Check sheet for the modelled part. Datum: model origin and axes. Units: mm. Face numbers are marked on the shaded views. Coordinates: 2 decimals unless noted, no trailing zeros. Loops run counter-clockwise (first coordinate to the right, second up) from the corner with the lowest first, then second, coordinate; pieces in that order, holes last. Notation, with made-up numbers: (1, -29) - (44, -29) arc R32 ccw to (44, 8) - close; hole circle Ø5 at (68, -31.75). An arc over 180 degrees is marked (long way). Write each question's results on one line, items separated by ' | '. Start each with the question number.
1. Cross-section at A-A (z = 7.5). Record the cut outline in (x, y).
2. Thickness scan on line 1 (Y direction, x = -18, z = 17.5); line 2 (X direction, y = 0, z = -17); line 3 (Y direction, x = 0, z = -17.5). Record the ranges inside material, lowest first. Write a range as [from, to].
3. Gauge pin test, flat ends, axial feed: P1, Ø3, axis at x = -26.5, y = -2.5, coming from the +Z side; P2, Ø4, axis at y = -2, z = -1, coming from the +X side. Record the tip position at first contact, or that the pin passes through.
4. Draft check along Y on the marked faces 1, 2, 3 and 4. Enter one of: released by +Y, released by -Y, zero draft, split by the parting line, or undercut.
5. Cross-section at C-C (z = -13). Record the cut outline in (x, y).
6. Cross-section at B-B (x = 14). Give the number of separate pieces and of enclosed holes in the cut face, and give its area (3 significant figures).
```python
from build123d import *

# Parameters (mm, degrees)
BOSS_EXTRUDE1_DEPTH     = 31
SKETCH2_R               = 18
BOSS_EXTRUDE2_DEPTH     = 1
SKETCH3_R               = 16
CUT_EXTRUDE1_DEPTH      = 73.520686704
CUT_EXTRUDE2_DEPTH      = 2
SKETCH5_R               = 3.5
CUT_EXTRUDE3_DEPTH      = 73.520686704
SKETCH6_W               = 3
SKETCH6_H               = 48
LPATTERN2_COUNT         = 9
LPATTERN2_PITCH         = 6
MIRROR1_COPY_1_SKETCH_W = 3
MIRROR1_COPY_1_SKETCH_H = 48
MIRROR1_COPY_2_SKETCH_W = 3
MIRROR1_COPY_2_SKETCH_H = 48
MIRROR1_COPY_3_SKETCH_W = 3
MIRROR1_COPY_3_SKETCH_H = 48
MIRROR1_COPY_4_SKETCH_W = 3
MIRROR1_COPY_4_SKETCH_H = 48
MIRROR1_COPY_5_SKETCH_W = 3
MIRROR1_COPY_5_SKETCH_H = 48
MIRROR1_COPY_6_SKETCH_W = 3
MIRROR1_COPY_6_SKETCH_H = 48
MIRROR1_COPY_7_SKETCH_W = 3
MIRROR1_COPY_7_SKETCH_H = 48
MIRROR1_COPY_8_SKETCH_W = 3
MIRROR1_COPY_8_SKETCH_H = 48
SKETCH8_W               = 48
SKETCH8_H               = 3
LPATTERN3_COUNT         = 9
LPATTERN3_PITCH         = 6
MIRROR2_COPY_1_SKETCH_W = 48
MIRROR2_COPY_1_SKETCH_H = 3
MIRROR2_COPY_2_SKETCH_W = 48
MIRROR2_COPY_2_SKETCH_H = 3
MIRROR2_COPY_3_SKETCH_W = 48
MIRROR2_COPY_3_SKETCH_H = 3
MIRROR2_COPY_4_SKETCH_W = 48
MIRROR2_COPY_4_SKETCH_H = 3
MIRROR2_COPY_5_SKETCH_W = 48
MIRROR2_COPY_5_SKETCH_H = 3
MIRROR2_COPY_6_SKETCH_W = 48
MIRROR2_COPY_6_SKETCH_H = 3
MIRROR2_COPY_7_SKETCH_W = 48
MIRROR2_COPY_7_SKETCH_H = 3
MIRROR2_COPY_8_SKETCH_W = 48
MIRROR2_COPY_8_SKETCH_H = 3


with BuildPart() as part:
    # Sketch1 → Boss-Extrude1 (new, symmetric)
    with BuildSketch(Plane.XY):
        with BuildLine():
            Line((18, 22.5), (-24, 22.5))
            ThreePointArc((-24, 22.5), (-26.828427125, 21.328427125), (-28, 18.5))
            Line((-28, 18.5), (-28, -18.5))
            ThreePointArc((-28, -18.5), (-26.828427125, -21.328427125), (-24, -22.5))
            Line((-24, -22.5), (18, -22.5))
            ThreePointArc((18, -22.5), (20.828427125, -21.328427125), (22, -18.5))
            Line((22, -18.5), (22, 18.5))
            ThreePointArc((22, 18.5), (20.828427125, 21.328427125), (18, 22.5))
        make_face()
    extrude(amount=BOSS_EXTRUDE1_DEPTH, both=True)

    # Sketch2 → Boss-Extrude2 (add, symmetric)
    with BuildSketch(Plane.XY.offset(31)):
        with Locations(Location((0, 0, 0), (0, 0, 180))):
            Circle(SKETCH2_R)
    extrude(amount=BOSS_EXTRUDE2_DEPTH, both=True)

    # Sketch3 → Cut-Extrude1 (cut, through all)
    with BuildSketch(Plane.XY.offset(32)):
        Circle(SKETCH3_R)
    extrude(amount=-CUT_EXTRUDE1_DEPTH, mode=Mode.SUBTRACT)

    # Sketch4 → Cut-Extrude2 (cut)
    with BuildSketch(Plane(origin=(0, 0, -31), x_dir=(-1, 0, 0), z_dir=(0, 0, -1))):
        with BuildLine():
            Line((12.872380115, 2), (12.872380115, -2))
            Line((12.872380115, -2), (22.61, -2))
            ThreePointArc((22.61, -2), (24.657927917, -0.354015138), (23.490928495, 2))
            Line((23.490928495, 2), (12.872380115, 2))
        make_face()
    extrude(amount=-CUT_EXTRUDE2_DEPTH, mode=Mode.SUBTRACT)

    # Sketch5 → Cut-Extrude3 (cut, through all)
    with BuildSketch(Plane(origin=(0, 0, -31), x_dir=(-1, 0, 0), z_dir=(0, 0, -1))):
        with Locations((-16.263455967, 16.263455967)):
            Circle(SKETCH5_R)
        with Locations((16.263455967, 16.263455967)):
            Circle(SKETCH5_R)
        with Locations((16.263455967, -16.263455967)):
            Circle(SKETCH5_R)
        with Locations((-16.263455967, -16.263455967)):
            Circle(SKETCH5_R)
    extrude(amount=-CUT_EXTRUDE3_DEPTH, mode=Mode.SUBTRACT)

    # Sketch6 → Cut-Revolve1 (revolve, cut)
    with BuildSketch(Plane(origin=(-3, 0, 0), x_dir=(0, 0, -1), z_dir=(1, 0, 0))):
        with Locations((25.5, 42.5)):
            Rectangle(SKETCH6_W, SKETCH6_H)
    cut_revolve1 = revolve(axis=Axis((-3, 66.5, -24), (0, 0, -1)), mode=Mode.SUBTRACT)

    # LPattern2: Cut-Revolve1 ×9
    with Locations(*[(0, 0, i * LPATTERN2_PITCH) for i in range(1, LPATTERN2_COUNT)]):
        add(cut_revolve1, mode=Mode.SUBTRACT)

    # Mirror1: Cut-Revolve1 across plane
    add(cut_revolve1.mirror(Plane.ZX), mode=Mode.SUBTRACT)

    # Mirror1 copy 1 sketch → Mirror1 copy 1 (revolve, cut)
    with BuildSketch(Plane(origin=(-3, 0, 6), x_dir=(0, 0, -1), z_dir=(1, 0, 0))):
        with Locations((25.5, -42.5)):
            Rectangle(MIRROR1_COPY_1_SKETCH_W, MIRROR1_COPY_1_SKETCH_H)
    revolve(axis=Axis((-3, -66.5, -18), (0, 0, 1)), mode=Mode.SUBTRACT)

    # Mirror1 copy 2 sketch → Mirror1 copy 2 (revolve, cut)
    with BuildSketch(Plane(origin=(-3, 0, 12), x_dir=(0, 0, -1), z_dir=(1, 0, 0))):
        with Locations((25.5, -42.5)):
            Rectangle(MIRROR1_COPY_2_SKETCH_W, MIRROR1_COPY_2_SKETCH_H)
    revolve(axis=Axis((-3, -66.5, -12), (0, 0, 1)), mode=Mode.SUBTRACT)

    # Mirror1 copy 3 sketch → Mirror1 copy 3 (revolve, cut)
    with BuildSketch(Plane(origin=(-3, 0, 18), x_dir=(0, 0, -1), z_dir=(1, 0, 0))):
        with Locations((25.5, -42.5)):
            Rectangle(MIRROR1_COPY_3_SKETCH_W, MIRROR1_COPY_3_SKETCH_H)
    revolve(axis=Axis((-3, -66.5, -6), (0, 0, 1)), mode=Mode.SUBTRACT)

    # Mirror1 copy 4 sketch → Mirror1 copy 4 (revolve, cut)
    with BuildSketch(Plane(origin=(-3, 0, 24), x_dir=(0, 0, -1), z_dir=(1, 0, 0))):
        with Locations((25.5, -42.5)):
            Rectangle(MIRROR1_COPY_4_SKETCH_W, MIRROR1_COPY_4_SKETCH_H)
    revolve(axis=Axis((-3, -66.5, 0), (0, 0, 1)), mode=Mode.SUBTRACT)

    # Mirror1 copy 5 sketch → Mirror1 copy 5 (revolve, cut)
    with BuildSketch(Plane(origin=(-3, 0, 30), x_dir=(0, 0, -1), z_dir=(1, 0, 0))):
        with Locations((25.5, -42.5)):
            Rectangle(MIRROR1_COPY_5_SKETCH_W, MIRROR1_COPY_5_SKETCH_H)
    revolve(axis=Axis((-3, -66.5, 6), (0, 0, 1)), mode=Mode.SUBTRACT)

    # Mirror1 copy 6 sketch → Mirror1 copy 6 (revolve, cut)
    with BuildSketch(Plane(origin=(-3, 0, 36), x_dir=(0, 0, -1), z_dir=(1, 0, 0))):
        with Locations((25.5, -42.5)):
            Rectangle(MIRROR1_COPY_6_SKETCH_W, MIRROR1_COPY_6_SKETCH_H)
    revolve(axis=Axis((-3, -66.5, 12), (0, 0, 1)), mode=Mode.SUBTRACT)

    # Mirror1 copy 7 sketch → Mirror1 copy 7 (revolve, cut)
    with BuildSketch(Plane(origin=(-3, 0, 42), x_dir=(0, 0, -1), z_dir=(1, 0, 0))):
        with Locations((25.5, -42.5)):
            Rectangle(MIRROR1_COPY_7_SKETCH_W, MIRROR1_COPY_7_SKETCH_H)
    revolve(axis=Axis((-3, -66.5, 18), (0, 0, 1)), mode=Mode.SUBTRACT)

    # Mirror1 copy 8 sketch → Mirror1 copy 8 (revolve, cut)
    with BuildSketch(Plane(origin=(-3, 0, 48), x_dir=(0, 0, -1), z_dir=(1, 0, 0))):
        with Locations((25.5, -42.5)):
            Rectangle(MIRROR1_COPY_8_SKETCH_W, MIRROR1_COPY_8_SKETCH_H)
    revolve(axis=Axis((-3, -66.5, 24), (0, 0, 1)), mode=Mode.SUBTRACT)

    # Sketch8 → Cut-Revolve2 (revolve, cut)
    with BuildSketch(Plane(origin=(0, 0, 0), x_dir=(1, 0, 0), z_dir=(0, 1, 0))):
        with Locations((-48, 25.5)):
            Rectangle(SKETCH8_W, SKETCH8_H)
    cut_revolve2 = revolve(axis=Axis((-72, 0, -27), (0, 0, 1)), mode=Mode.SUBTRACT)

    # LPattern3: Cut-Revolve2 ×9
    with Locations(*[(0, 0, i * LPATTERN3_PITCH) for i in range(1, LPATTERN3_COUNT)]):
        add(cut_revolve2, mode=Mode.SUBTRACT)

    # Mirror2: Cut-Revolve2 across plane
    add(cut_revolve2.mirror(Plane(origin=(-3, 0, 0), x_dir=(0, 0, 1), z_dir=(1, 0, 0))), mode=Mode.SUBTRACT)

    # Mirror2 copy 1 sketch → Mirror2 copy 1 (revolve, cut)
    with BuildSketch(Plane(origin=(-6, 0, 6), x_dir=(-1, 0, 0), z_dir=(0, 1, 0))):
        with Locations((-48, -25.5)):
            Rectangle(MIRROR2_COPY_1_SKETCH_W, MIRROR2_COPY_1_SKETCH_H)
    revolve(axis=Axis((66, 0, -21), (0, 0, -1)), mode=Mode.SUBTRACT)

    # Mirror2 copy 2 sketch → Mirror2 copy 2 (revolve, cut)
    with BuildSketch(Plane(origin=(-6, 0, 12), x_dir=(-1, 0, 0), z_dir=(0, 1, 0))):
        with Locations((-48, -25.5)):
            Rectangle(MIRROR2_COPY_2_SKETCH_W, MIRROR2_COPY_2_SKETCH_H)
    revolve(axis=Axis((66, 0, -15), (0, 0, -1)), mode=Mode.SUBTRACT)

    # Mirror2 copy 3 sketch → Mirror2 copy 3 (revolve, cut)
    with BuildSketch(Plane(origin=(-6, 0, 18), x_dir=(-1, 0, 0), z_dir=(0, 1, 0))):
        with Locations((-48, -25.5)):
            Rectangle(MIRROR2_COPY_3_SKETCH_W, MIRROR2_COPY_3_SKETCH_H)
    revolve(axis=Axis((66, 0, -9), (0, 0, -1)), mode=Mode.SUBTRACT)

    # Mirror2 copy 4 sketch → Mirror2 copy 4 (revolve, cut)
    with BuildSketch(Plane(origin=(-6, 0, 24), x_dir=(-1, 0, 0), z_dir=(0, 1, 0))):
        with Locations((-48, -25.5)):
            Rectangle(MIRROR2_COPY_4_SKETCH_W, MIRROR2_COPY_4_SKETCH_H)
    revolve(axis=Axis((66, 0, -3), (0, 0, -1)), mode=Mode.SUBTRACT)

    # Mirror2 copy 5 sketch → Mirror2 copy 5 (revolve, cut)
    with BuildSketch(Plane(origin=(-6, 0, 30), x_dir=(-1, 0, 0), z_dir=(0, 1, 0))):
        with Locations((-48, -25.5)):
            Rectangle(MIRROR2_COPY_5_SKETCH_W, MIRROR2_COPY_5_SKETCH_H)
    revolve(axis=Axis((66, 0, 3), (0, 0, -1)), mode=Mode.SUBTRACT)

    # Mirror2 copy 6 sketch → Mirror2 copy 6 (revolve, cut)
    with BuildSketch(Plane(origin=(-6, 0, 36), x_dir=(-1, 0, 0), z_dir=(0, 1, 0))):
        with Locations((-48, -25.5)):
            Rectangle(MIRROR2_COPY_6_SKETCH_W, MIRROR2_COPY_6_SKETCH_H)
    revolve(axis=Axis((66, 0, 9), (0, 0, -1)), mode=Mode.SUBTRACT)

    # Mirror2 copy 7 sketch → Mirror2 copy 7 (revolve, cut)
    with BuildSketch(Plane(origin=(-6, 0, 42), x_dir=(-1, 0, 0), z_dir=(0, 1, 0))):
        with Locations((-48, -25.5)):
            Rectangle(MIRROR2_COPY_7_SKETCH_W, MIRROR2_COPY_7_SKETCH_H)
    revolve(axis=Axis((66, 0, 15), (0, 0, -1)), mode=Mode.SUBTRACT)

    # Mirror2 copy 8 sketch → Mirror2 copy 8 (revolve, cut)
    with BuildSketch(Plane(origin=(-6, 0, 48), x_dir=(-1, 0, 0), z_dir=(0, 1, 0))):
        with Locations((-48, -25.5)):
            Rectangle(MIRROR2_COPY_8_SKETCH_W, MIRROR2_COPY_8_SKETCH_H)
    revolve(axis=Axis((66, 0, 21), (0, 0, -1)), mode=Mode.SUBTRACT)


solid = part.part
```
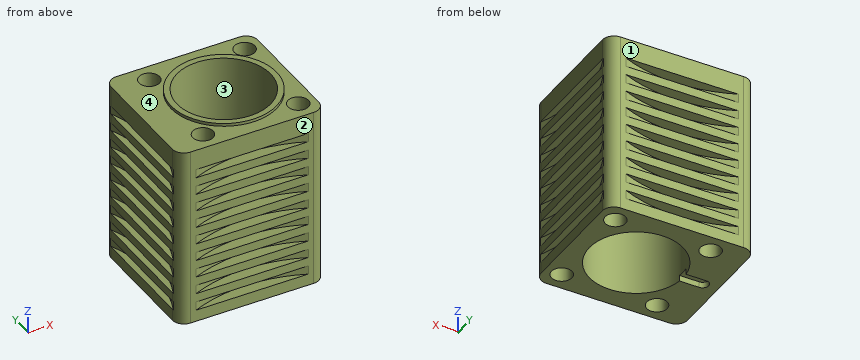
Established:
1) outline: (-28, -18.5) arc R4 ccw to (-24, -22.5) - (18, -22.5) arc R4 ccw to (22, -18.5) - (22, 18.5) arc R4 ccw to (18, 22.5) - (-24, 22.5) arc R4 ccw to (-28, 18.5) - close; hole circle Ø7 at (-16.26, -16.26); hole circle Ø7 at (-16.26, 16.26); hole circle Ø32 at (0, 0); hole circle Ø7 at (16.26, -16.26); hole circle Ø7 at (16.26, 16.26)
2) line 1: [-20.9, -19.3], [-13.22, 13.22], [19.3, 20.9] | line 2: [-28, -16], [16, 22] | line 3: [-22.5, -16], [16, 22.5]
3) P1: z = 31 | P2: x = 22
4) face 1: released by +Y | face 2: released by -Y | face 3: undercut | face 4: zero draft
5) outline: (-27.96, -19.08) arc R4 ccw to (-24, -22.5) - (-22.18, -22.5) arc R48 cw to (16.18, -22.5) - (18, -22.5) arc R4 ccw to (21.96, -19.08) arc R48 cw to (21.96, 19.08) arc R4 ccw to (18, 22.5) - (16.18, 22.5) arc R48 cw to (-22.18, 22.5) - (-24, 22.5) arc R4 ccw to (-27.96, 19.08) arc R48 cw to start; hole circle Ø7 at (-16.26, -16.26); hole circle Ø7 at (-16.26, 16.26); hole circle Ø32 at (0, 0); hole circle Ø7 at (16.26, -16.26); hole circle Ø7 at (16.26, 16.26)
6) separate pieces: 4 | enclosed holes: 0 | area: 1,130 mm^2
